The listing builds one solid part. Answer for the finished solid, in the listing's coordinates (mm). A direction names the side the tool comes from. Coordinates: 2 decimals unless noted, no trailing zeros. Write each loop counter-clockwise with the first axis right and the second up, starting at its lowest first coordinate (ties: lowest second). Pieces come first, ordered by that corner, then holes. Notation, with made-up numbers: M -31,73.25 L -9,73.25 A34 cw -9,106.25 Z; hole C -37.5,89.25 d11. An arc over 180 degrees is marked long. Put each result on its own line as item: value. Start each with the question number.
Autodesk Inventor part; units mm, degrees
ref_plane "YZ Plane" through (0, 0, 0) normal (1, 0, 0) x (0, 1, 0)
ref_plane "XZ Plane" through (0, 0, 0) normal (0, 1, 0) x (-1, 0, 0)
ref_plane "XY Plane" through (0, 0, 0) normal (0, 0, 1) x (1, 0, 0)
sketch "スケッチ1" plane through (0, 0, 0) normal (0, 0, 1) x (1, 0, 0)
  line L0 (0, 0) -> (10, 0)
  line L1 (10, 0) -> (10, 10)
  line L2 (10, 10) -> (0, 10)
  line L3 (0, 10) -> (0, 0)
  line L4 (1, 9) -> (9, 9)
  line L5 (9, 9) -> (9, 1)
  line L6 (9, 1) -> (1, 1)
  line L7 (1, 1) -> (1, 9)
  dimension "d0" = 10
  dimension "d1" = 10
  dimension "d2" = 1
extrude "押し出し1" add sketch "スケッチ1" along normal blind 20
sketch "スケッチ2" plane through (10, 0, 0) normal (1, 0, 0) x (0, 0, -1)
  line L0 (-20, 0) -> (-20, 10)
  point P0 (0, 0)
  point P1 (-16, 5)
  dimension "d5" = 4
hole "穴1" at (10, 5, 16) direction (-1, 0, 0) diameter 4 end through all
sketch "スケッチ3" plane through (0, 10, 0) normal (0, 1, 0) x (1, 0, 0)
  line L0 (10, -20) -> (0, -20)
  point P0 (0, 0)
  point P1 (5, -6)
  dimension "d13" = 14
hole "穴2" at (5, 10, 6) direction (0, -1, 0) diameter 6 end through all
properties part number "finger_k_mk_1"
1) A cutting plane is placed at C-C on y = 5. Write down the section's boundary in (x, z), then the cut area to 3 significant figures.
2) For faces 1 (the face through (1, 5, 10)), 2 (the face through (0.5, 5.1, 20)), determine the directions among +Z, -Z, +X, -X, +Y, -Y from which every point of the face is accessible in a straight line to the end or side of a thin tool.
3) Straight lines are drawn through the part: probe 1 along Y at (x, z) = (6.5, 17.5); probe 2 along Z at (x, y) = (5, 9.2); probe 3 along Y at (x, z) = (0.35, 16). For each, find the intervals that lie inside material, in ascending order.
4) A cutting plane is placed at A-A on z = 6. Write down the section's boundary in (x, y).
5) Determine the mould class of faces 3 (the face through (0.5, 5.1, 0)), 4 (the face through (5, 1, 10)), 5 (the face through (0.5, 6.2, 17.6)) for opening direction Z: +Z half, -Z half, draft (parallel to the pull), parting line (faces both ways), or undercut.
6) A cutting plane is placed at B-B on y = 7.75. Write down the section's boundary in (x, z).
Answers follow:
1. outline: M 0,0 L 1,0 L 1,14 L 0,14 Z; M 0,18 L 1,18 L 1,20 L 0,20 Z; M 9,0 L 10,0 L 10,14 L 9,14 Z; M 9,18 L 10,18 L 10,20 L 9,20 Z
1. area: 32.0 mm²
2. face 1: +Z, -Z
2. face 2: +Z, +X, -X, +Y, -Y
3. probe 1: y = 0 to 1, 9 to 10
3. probe 2: z = 0 to 3, 9 to 20
3. probe 3: y = 0 to 3, 7 to 10
4. outline: M 0,0 L 2,0 L 2,1 L 1,1 L 1,9 L 2,9 L 2,10 L 0,10 Z; M 8,0 L 10,0 L 10,10 L 8,10 L 8,9 L 9,9 L 9,1 L 8,1 Z
5. face 3: -Z half
5. face 4: draft
5. face 5: undercut
6. outline: M 0,0 L 1,0 L 1,20 L 0,20 Z; M 9,0 L 10,0 L 10,20 L 9,20 Z
